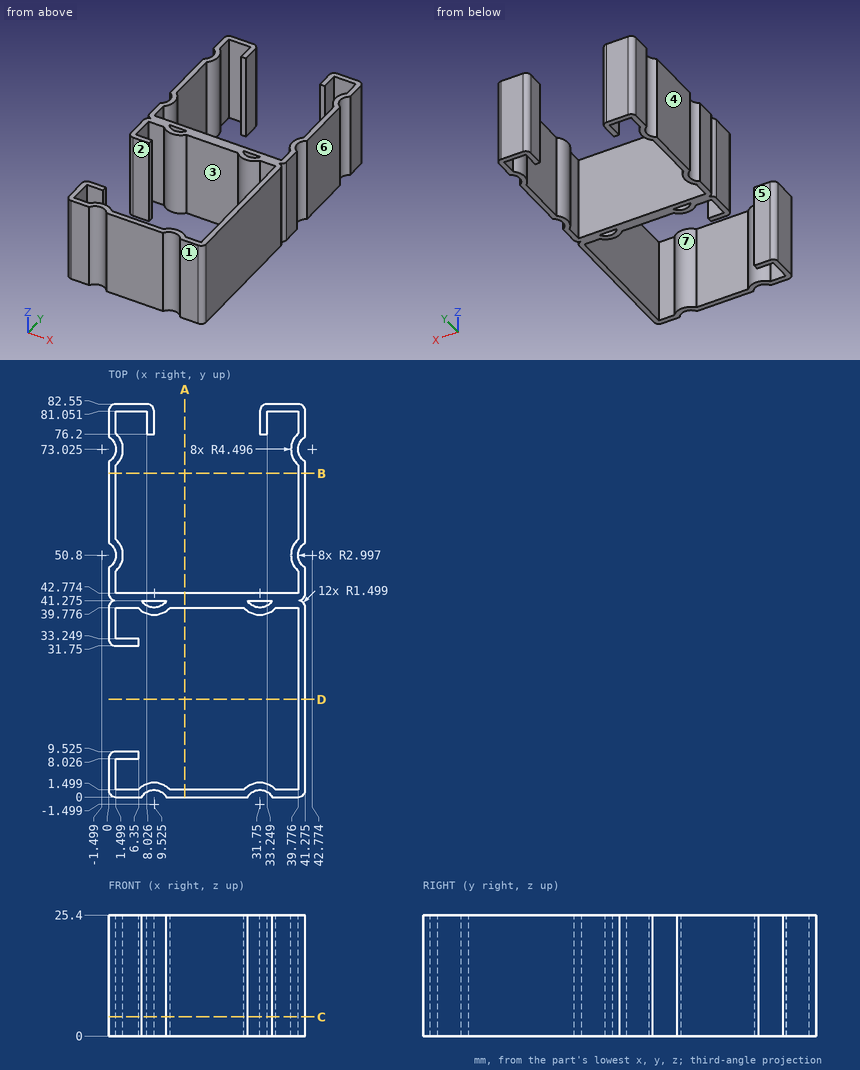
Geometry check sheet. Reference: drawing and pictorial views, mm from the part's lowest x, y, z. A direction names the side the tool comes from. Round coordinates to 2 decimals unless told otherwise and drop trailing zeros. Loops run counter-clockwise (first coordinate to the right, second up) from the corner with the lowest first, then second, coordinate; pieces in that order, holes last. Notation, with made-up numbers: (-16, 23.5) - (-2, 23.5) arc R32 ccw to (-2, 55.5) - close; hole circle Ø11 at (11.5, -12). An arc over 180 degrees is marked (long way). Write item = value, one per line. Start each with the question number.
Q1. Access from +Z, -Z, +X, -X, +Y, -Y to the whole of each face (thin tool, end or side, straight path). Record for the marked faces 1, 2 and 3.
Q2. Section check B-B (y = 68). Record the boundary of the cut face in (x, z) (1 decimal).
Q3. Depth check by flat-ended pin: P1, Ø2, axis at x = 8.5, z = 12.5, coming from the -Y side; P2, Ø1, axis at x = 33.5, z = 20.5, coming from the -Y side; P3, Ø2, axis at x = 10.5, z = 3, coming from the -Y side (1 decimal); P4, Ø12, axis at x = 21.5, y = 73.5, coming from the +Z side. Enter the tip coordinate at first touch or a pass-through.
Q4. Section check D-D (y = 20.5). Record the boundary of the cut face in (x, z) (1 decimal).
Q5. Section check A-A (x = 16). Record the boundary of the cut face in (y, z), plus the area to 3 significant figures.
Q6. Release check for a two-part mould opening along X. For the marked faces 4, 5, 6 and 7 record: pulls with the +X half, pulls with the -X half, needs draft (parallel to the pull), parting line crosses it, or undercut.
Q7. Thickness scan on L1, parallel to Y at x = 36.5, z = 20; L2, parallel to Y at x = 31.5, z = 21 (1 decimal); L3, parallel to Y at x = 16, z = 24.25. Record the ranges inside material, lowest first.
Q8. Section check C-C (z = 4). Count the separate pieces of the cut face and the enclosed holes in it.
Derived:
q1.face_1 = +Z, -Z, +X, -X, -Y
q1.face_2 = +Z, -Z, -X
q1.face_3 = +Z, -Z
q2.outline = (0, 0) - (1.5, 0) - (1.5, 25.4) - (0, 25.4) - close; (39.8, 0) - (41.3, 0) - (41.3, 25.4) - (39.8, 25.4) - close
q3.P1 = 0.71
q3.P2 = 0.48
q3.P3 = 0.8
q3.P4 = through
q4.outline = (39.8, 0) - (41.3, 0) - (41.3, 25.4) - (39.8, 25.4) - close
q5.outline = (0, 0) - (1.5, 0) - (1.5, 25.4) - (0, 25.4) - close; (39.78, 0) - (42.77, 0) - (42.77, 25.4) - (39.78, 25.4) - close
q5.area = 114 mm^2
q6.face_4 = pulls with the -X half
q6.face_5 = needs draft
q6.face_6 = pulls with the +X half
q6.face_7 = undercut
q7.L1 = 0 to 1.5, 39.78 to 42.77, 81.05 to 82.55
q7.L2 = 1.5 to 3, 38.3 to 39.8, 41.3 to 42.8
q7.L3 = 0 to 1.5, 39.78 to 42.77
q8.separate_pieces = 1
q8.enclosed_holes = 2
